```python
from build123d import *

# Parameters (mm, degrees)
F0_R     = 20.32
F0_R_2   = 17.526
F1_DEPTH = 38.1
F2_W     = 53.34
F2_H     = 53.34
F3_DEPTH = 3.175
F4_R     = 7.14375
F5_DEPTH = 12.7


with BuildPart() as f1:
    # F0 (on Top) → F1 (new body)
    with BuildSketch(Plane.XY):
        Circle(F0_R)
        Circle(F0_R_2, mode=Mode.SUBTRACT)
    extrude(amount=F1_DEPTH)

    # F2 (on Top) → F3 (join)
    with BuildSketch(Plane.XY):
        Rectangle(F2_W, F2_H)
    extrude(amount=F3_DEPTH)

    # F4 (on face) → F5 (join)
    with BuildSketch(Plane.XY.offset(3.175)):
        Circle(F4_R)
    extrude(amount=F5_DEPTH)


solid = f1.part
```
The listing builds one solid part. Answer for the finished solid, in the listing's coordinates (mm). A direction names the side the tool comes from. Coordinates: 2 decimals unless noted, no trailing zeros. Write each loop counter-clockwise with the first axis right and the second up, starting at its lowest first coordinate (ties: lowest second). Pieces come first, ordered by that corner, then holes. Notation, with made-up numbers: (36.25, 7.25) -> (60.25, 7.25) arc R31 cw to (60.25, 38.25) -> close; hole circle Ø2 at (-7, -0.75). An arc over 180 degrees is marked (long way). Write each question's results on one line, items separated by ' | '. Start each with the question number.
1) A cutting plane is placed at D-D (z = 28). Determine the outline of the cut face in (x, y).
2) A tool of negligible diameter and unlimited length cuts with its end or side. For faces 4 (the cylindrical face through (-2.645, 20.147, 20.393)), 5 (the flat face through (0, -26.67, 2)), from which of +Z, -Z, +X, -X, +Y, -Y can it reach the whole face along a straight path? Write none if from no direction.
3) A cutting plane is placed at B-B (y = 0). Determine the outline of the cut face in (x, z) (3 decimals).
4) Flat-ended cylindrical pins translate along their axes: pin 1 Ø6 at (x, y) = (1, 8.5) entering from +Z (3 decimals); pin 2 Ø10 at (y, z) = (6.5, 13) entering from -X; pin 3 Ø4 at (y, z) = (18, 13) entering from +X. Find the tip coordinate at first contact, or state that the pin passes through.
5) A cutting plane is placed at A-A (z = 6). Determine the outline of the cut face in (x, y), then the cut area to 3 significant figures.
6) Straight lines are drawn through the part: probe 1 along Y at (x, z) = (0, 11); probe 2 along Y at (x, z) = (0, 23); probe 3 along Y at (x, z) = (5.5, 6). For each, find the intervals that lie inside material, in ascending order.
7) For a pull along X with two mould halves and no side action, classify faces 1 (the cylindrical face through (-7.137, 0.314, 9.436)), 2 (the flat face through (-17, -6, 38.1)), 3 (the flat face through (26.67, 0, 2)) as +X half, -X half, draft (parallel to the pull), parting line (faces both ways), or undercut.
Values follow:
1) outline: circle Ø40.64 at (0, 0); hole circle Ø35.05 at (0, 0)
2) face 4: +Z | face 5: +Z, -Z, +X, -X, -Y
3) outline: (-26.67, 0) -> (26.67, 0) -> (26.67, 3.175) -> (20.32, 3.175) -> (20.32, 38.1) -> (17.526, 38.1) -> (17.526, 3.175) -> (7.144, 3.175) -> (7.144, 15.875) -> (-7.144, 15.875) -> (-7.144, 3.175) -> (-17.526, 3.175) -> (-17.526, 38.1) -> (-20.32, 38.1) -> (-20.32, 3.175) -> (-26.67, 3.175) -> close
4) pin 1: z = 15.875 | pin 2: x = -20.26 | pin 3: x = 12.53
5) outline: circle Ø40.64 at (0, 0); circle Ø14.29 at (0, 0); hole circle Ø35.05 at (0, 0) | area: 493 mm²
6) probe 1: -20.32 to -17.53, -7.14 to 7.14, 17.53 to 20.32 | probe 2: -20.32 to -17.53, 17.53 to 20.32 | probe 3: -19.56 to -16.64, -4.56 to 4.56, 16.64 to 19.56
7) face 1: undercut | face 2: draft | face 3: +X half
